Work out the finished part from the listing and answer in its coordinate system (mm). Face numbers are marked on the shaded views. A direction names the side the tool comes from. Coordinates: 2 decimals unless noted, no trailing zeros. Write each loop counter-clockwise with the first axis right and the second up, starting at its lowest first coordinate (ties: lowest second). Pieces come first, ordered by that corner, then holes. Notation, with made-up numbers: (39.25, -7) - (86.25, -7) arc R14 cw to (86.25, 8) - close; hole circle Ø11 at (16, 16.25). An arc over 180 degrees is marked (long way). Use one line per item in the form item = value. Start each with the question number.
Item 1: A cutting plane is placed at A-A (z = -3.2). Write down the section's boundary in (x, y), then the cut area to 3 significant figures.
Item 2: A cutting plane is placed at B-B (x = 11.5). Write down the section's boundary in (y, z).
Item 3: A cutting plane is placed at D-D (x = 5.25). Write down the section's boundary in (y, z), then the cut area to 3 significant figures.
Item 4: For the marked faces 4, 5 and 6, determine the directions among +Z, -Z, +X, -X, +Y, -Y from which every point of the face is accessible in a straight line to the end or side of a thin tool.
Item 5: Consider probe 1 along X at (y, z) = (1.85, -13.8); probe 2 along Z at (x, y) = (7.75, 0.95); probe 3 along Z at (x, y) = (5.25, 0.45). Determine where each line is inside the solid, lowest interval first.
Item 6: Given pin 1 (4.5 mm diameter, centred on x = 5.25, z = -13.8, fed in from -Y); pin 2 (1.6 mm diameter, centred on x = 4, z = -14, fed in from +Y); pin 3 (0.6 mm diameter, centred on x = 4.5, z = -9, fed in from -Y); pin 4 (2.5 mm diameter, centred on x = 5.25, z = -3.2, fed in from -Y), each flat-ended and moving along its own axis, determine where each tip first touches the part or whether it passes through.
Item 7: A cutting plane is placed at C-C (y = 2). Write down the section's boundary in (x, z).
Item 8: Determine the mould class of the marked faces 1, 2 and 3 for opening direction X: released by +X, released by -X, zero draft, split by the parting line, or undercut.
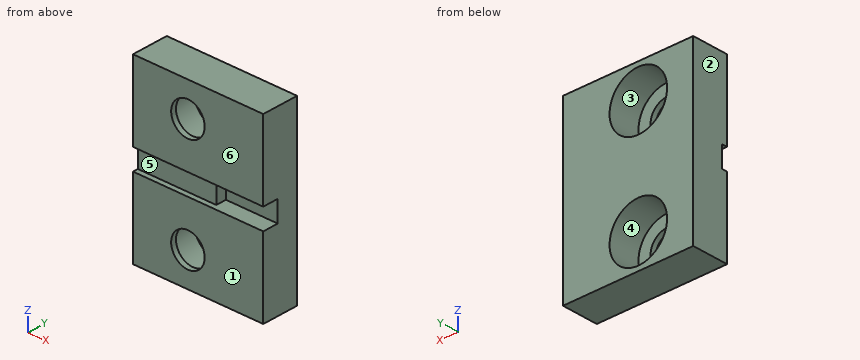
from build123d import *

# Parameters (mm, degrees)
CROQUIS1_W              = 10.5
CROQUIS1_H              = 17
CROQUIS1_R              = 1.6
SALIENTE_EXTRUIR1_DEPTH = 3.5
CROQUIS2_R              = 2.75
CORTAR_EXTRUIR1_DEPTH   = 3
CROQUIS3_W              = 2
CROQUIS3_H              = 0.5
CORTAR_EXTRUIR2_DEPTH   = 16
CROQUIS4_W              = 3
CROQUIS4_H              = 2
CORTAR_EXTRUIR3_DEPTH   = 1
SALIENTE_EXTRUIR2_DEPTH = 10
CROQUIS6_W              = 8.05
CROQUIS6_H              = 17
CORTAR_EXTRUIR4_DEPTH   = 10


with BuildPart() as part:
    # Croquis1 → Saliente-Extruir1 (new body)
    with BuildSketch(Plane(origin=(0, 0, 0), x_dir=(1, 0, 0), z_dir=(0, 1, 0))):
        with Locations((5.25, 8.5)):
            Rectangle(CROQUIS1_W, CROQUIS1_H)
        with Locations(Location((5.25, 13.8, 0), (0, 0, 270))):
            Circle(CROQUIS1_R, mode=Mode.SUBTRACT)
        with Locations(Location((5.25, 3.2, 0), (0, 0, 90))):
            Circle(CROQUIS1_R, mode=Mode.SUBTRACT)
    extrude(amount=SALIENTE_EXTRUIR1_DEPTH)

    # Croquis2 → Cortar-Extruir1 (cut)
    with BuildSketch(Plane(origin=(0, 3.5, 0), x_dir=(1, 0, 0), z_dir=(0, 1, 0))):
        with Locations(Location((5.25, 13.8, 0), (0, 0, 270))):
            Circle(CROQUIS2_R)
        with Locations(Location((5.25, 3.2, 0), (0, 0, 270))):
            Circle(CROQUIS2_R)
    extrude(amount=-CORTAR_EXTRUIR1_DEPTH, mode=Mode.SUBTRACT)

    # Croquis3 → Cortar-Extruir2 (cut)
    with BuildSketch(Plane(origin=(10.5, 0, 0), x_dir=(0, 0, -1), z_dir=(1, 0, 0))):
        with Locations((8.5, 0.25)):
            Rectangle(CROQUIS3_W, CROQUIS3_H)
    extrude(amount=-CORTAR_EXTRUIR2_DEPTH, mode=Mode.SUBTRACT)

    # Croquis4 → Cortar-Extruir3 (cut)
    with BuildSketch(Plane.XZ.offset(-0.5)):
        with Locations((9, -8.5)):
            Rectangle(CROQUIS4_W, CROQUIS4_H)
    extrude(amount=-CORTAR_EXTRUIR3_DEPTH, mode=Mode.SUBTRACT)

    # Croquis5 → Saliente-Extruir2 (add)
    with BuildSketch(Plane(origin=(10.5, 0, 0), x_dir=(0, 0, -1), z_dir=(1, 0, 0))):
        Polygon((7.5, 1.5), (9.5, 1.5), (9.5, 0), (17, 0), (17, 3.5), (0, 3.5), (0, 0), (7.5, 0), align=None)
    extrude(amount=SALIENTE_EXTRUIR2_DEPTH)

    # Croquis6 → Cortar-Extruir4 (cut)
    with BuildSketch(Plane(origin=(0, 3.5, 0), x_dir=(1, 0, 0), z_dir=(0, 1, 0))):
        with Locations((16.475, 8.5)):
            Rectangle(CROQUIS6_W, CROQUIS6_H)
    extrude(amount=-CORTAR_EXTRUIR4_DEPTH, mode=Mode.SUBTRACT)


solid = part.part
Answer:
q1.outline = (0, 0) - (3.65, 0) - (3.65, 0.5) - (2.5, 0.5) - (2.5, 3.5) - (0, 3.5) - close; (6.85, 0) - (12.45, 0) - (12.45, 3.5) - (8, 3.5) - (8, 0.5) - (6.85, 0.5) - close
q1.area = 25.5 mm²
q2.outline = (0, -17) - (3.5, -17) - (3.5, 0) - (0, 0) - (0, -7.5) - (1.5, -7.5) - (1.5, -9.5) - (0, -9.5) - close
q3.outline = (0, -17) - (3.5, -17) - (3.5, -16.55) - (0.5, -16.55) - (0.5, -15.4) - (0, -15.4) - close; (0, -12.2) - (0.5, -12.2) - (0.5, -11.05) - (3.5, -11.05) - (3.5, -5.95) - (0.5, -5.95) - (0.5, -4.8) - (0, -4.8) - (0, -7.5) - (0.5, -7.5) - (0.5, -9.5) - (0, -9.5) - close; (0, -1.6) - (0.5, -1.6) - (0.5, -0.45) - (3.5, -0.45) - (3.5, 0) - (0, 0) - close
q3.area = 22.3 mm²
q4.face_4 = +Y
q4.face_5 = +X, -X, -Y
q4.face_6 = +Z, -Z, +X, -X, -Y
q5.probe_1 = 0 to 2.5, 8 to 12.45
q5.probe_2 = -17 to -14.95, -12.65 to -9.5, -7.5 to -4.35, -2.05 to 0
q5.probe_3 = -17 to -15.4, -12.2 to -9.5, -7.5 to -4.8, -1.6 to 0
q6.pin_1 = 0
q6.pin_2 = 0.5
q6.pin_3 = 0.5
q6.pin_4 = through
q7.outline = (0, -17) - (12.45, -17) - (12.45, 0) - (0, 0) - close; hole circle Ø5.5 at (5.25, -13.8); hole circle Ø5.5 at (5.25, -3.2)
q8.face_1 = zero draft
q8.face_2 = released by -X
q8.face_3 = undercut
